Geometry: final body of the model. Coordinates: model frame, mm. Face numbers are marked on the shaded views. A direction names the side the tool comes from. Round coordinates to 2 decimals unless told otherwise and drop trailing zeros. Loops run counter-clockwise (first coordinate to the right, second up) from the corner with the lowest first, then second, coordinate; pieces in that order, holes last. Notation, with made-up numbers: M -37,-19.75 L -27,-19.75 A18 cw -27,15.25 Z; hole C 67.5,74 d8. An arc over 180 degrees is marked long. Answer as a JSON object with one key per item and string values.
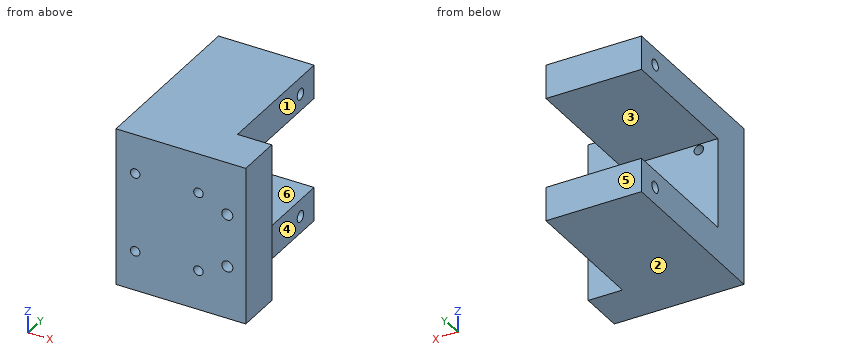
from build123d import *

# Parameters (mm, degrees)
CROQUIS1_R              = 1.8
CROQUIS1_R_2            = 2.1
SALIENTE_EXTRUIR4_DEPTH = 17
CROQUIS2_W              = 48.25
CROQUIS2_H              = 10
SALIENTE_EXTRUIR5_DEPTH = 17
CROQUIS3_W              = 36.25
CROQUIS3_H              = 12.86
SALIENTE_EXTRUIR6_DEPTH = 50
CROQUIS4_R              = 2.1
CORTAR_EXTRUIR1_DEPTH   = 50
CROQUIS5_W              = 60
CROQUIS5_H              = 17
SALIENTE_EXTRUIR7_DEPTH = 1


with BuildPart() as part:
    # Croquis1 → Saliente-Extruir4 (new body)
    with BuildSketch(Plane(origin=(0, 0, 0), x_dir=(1, 0, 0), z_dir=(0, 1, 0))):
        Polygon((0, 0), (48.11, 0), (48.25, 0), (48.25, 20), (48.25, 40), (48.11, 40), (0, 40), align=None)
        with Locations((7.3, 5)):
            Circle(CROQUIS1_R, mode=Mode.SUBTRACT)
        with Locations((31.3, 5)):
            Circle(CROQUIS1_R, mode=Mode.SUBTRACT)
        with Locations((31.3, 35)):
            Circle(CROQUIS1_R, mode=Mode.SUBTRACT)
        with Locations((7.3, 35)):
            Circle(CROQUIS1_R, mode=Mode.SUBTRACT)
        with Locations((42.25, 30)):
            Circle(CROQUIS1_R_2, mode=Mode.SUBTRACT)
        with Locations((42.25, 10)):
            Circle(CROQUIS1_R_2, mode=Mode.SUBTRACT)
    extrude(amount=SALIENTE_EXTRUIR4_DEPTH)

    # Croquis2 → Saliente-Extruir5 (add)
    with BuildSketch(Plane(origin=(0, 17, 0), x_dir=(1, 0, 0), z_dir=(0, 1, 0))):
        with Locations((24.125, 45)):
            Rectangle(CROQUIS2_W, CROQUIS2_H)
        with Locations((24.125, -5)):
            Rectangle(CROQUIS2_W, CROQUIS2_H)
    extrude(amount=-SALIENTE_EXTRUIR5_DEPTH)

    # Croquis3 → Saliente-Extruir6 (add)
    with BuildSketch(Plane(origin=(0, 17, 0), x_dir=(1, 0, 0), z_dir=(0, 1, 0))):
        with Locations((18.125, 43.57)):
            Rectangle(CROQUIS3_W, CROQUIS3_H)
        with Locations((18.125, -3.57)):
            Rectangle(CROQUIS3_W, CROQUIS3_H)
    extrude(amount=SALIENTE_EXTRUIR6_DEPTH)

    # Croquis4 → Cortar-Extruir1 (cut)
    with BuildSketch(Plane.ZY):
        with Locations((-43.57, 58.1)):
            Circle(CROQUIS4_R)
        with Locations((3.57, 58.1)):
            Circle(CROQUIS4_R)
    extrude(amount=-CORTAR_EXTRUIR1_DEPTH, mode=Mode.SUBTRACT)

    # Croquis5 → Saliente-Extruir7 (add)
    with BuildSketch(Plane(origin=(48.25, 0, 0), x_dir=(0, 0, -1), z_dir=(1, 0, 0))):
        with Locations((20, 8.5)):
            Rectangle(CROQUIS5_W, CROQUIS5_H)
    extrude(amount=SALIENTE_EXTRUIR7_DEPTH)


solid = part.part
1) Section query C-C (y = 21). Return the cut outline in (x, z).
Results:
{"outline": "M 0,-50 L 36.25,-50 L 36.25,-37.14 L 0,-37.14 Z; M 0,-2.86 L 36.25,-2.86 L 36.25,10 L 0,10 Z"}
2) Section query A-A (x = 7.3). Return the cut outline in (y, z).
Results:
{"outline": "M 0,-50 L 67,-50 L 67,-37.14 L 17,-37.14 L 17,-36.8 L 0,-36.8 Z; M 0,-33.2 L 17,-33.2 L 17,-6.8 L 0,-6.8 Z; M 0,-3.2 L 17,-3.2 L 17,-2.86 L 67,-2.86 L 67,10 L 0,10 Z; hole C 58.1,-43.57 d4.2; hole C 58.1,3.57 d4.2"}
3) Pull-direction query (Z, two-part tool) for the marked faces 1, 2 and 3; classes: +Z half, -Z half, draft (parallel to the pull), parting line (faces both ways), or undercut.
Results:
{"face 1": "draft", "face 2": "-Z half", "face 3": "undercut"}
4) Pin query (flat end, axial travel): P1, Ø6, axis at y = 15, z = -27, coming from the -X side; P2, Ø3, axis at x = 31.3, z = -5, coming from the +Y side; P3, Ø10.5, axis at y = 34, z = 4, coming from the +X side; P4, Ø10, axis at x = 27.5, z = -28, coming from the +Y side. Return the tip coordinate at first contact, or that it passes through.
Results:
{"P1": "x = 0", "P2": "through", "P3": "x = 36.25", "P4": "y = 17"}
5) Section query B-B (z = -35). Return the cut outline in (x, y).
Results:
{"outline": "M 0,0 L 5.5,0 L 5.5,17 L 0,17 Z; M 9.1,0 L 29.5,0 L 29.5,17 L 9.1,17 Z; M 33.1,0 L 49.25,0 L 49.25,17 L 33.1,17 Z"}
6) Ray query, line 1 (Z direction, x = 7.3, y = 5); line 2 (X direction, y = 4, z = -5); line 3 (Z direction, x = 42, y = 6). Return the intervals inside material, ascending.
Results:
{"line 1": "-50 to -36.8, -33.2 to -6.8, -3.2 to 10", "line 2": "0 to 5.5, 9.1 to 29.5, 33.1 to 49.25", "line 3": "-50 to -32.09, -27.91 to -12.09, -7.91 to 10"}
7) Reachability of the marked faces 4, 5 and 6 from +Z, -Z, +X, -X, +Y, -Y: full face, straight path, thin tool, end or side. Return the list, or none.
Results:
{"face 4": "+Z, -Z, +X, +Y", "face 5": "+Z, -Z, +X, -X, +Y", "face 6": "+X, -X, +Y"}
8) Section query D-D (y = 58.1). Return the cut outline in (x, z), and give its area (3 significant figures).
Results:
{"outline": "M 0,-50 L 36.25,-50 L 36.25,-45.67 L 0,-45.67 Z; M 0,-41.47 L 36.25,-41.47 L 36.25,-37.14 L 0,-37.14 Z; M 0,-2.86 L 36.25,-2.86 L 36.25,1.47 L 0,1.47 Z; M 0,5.67 L 36.25,5.67 L 36.25,10 L 0,10 Z", "area": "628 mm2"}
